CAD build for the part. Positions are in the model's coordinates, mm. Face numbers are marked on the shaded views. Round coordinates to 2 decimals unless told otherwise and drop trailing zeros. Loops run counter-clockwise (first coordinate to the right, second up) from the corner with the lowest first, then second, coordinate; pieces in that order, holes last.
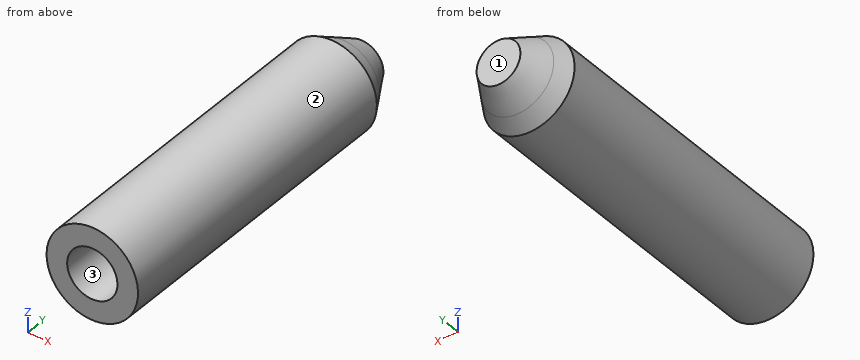
from build123d import *


with BuildPart() as f1:
    # F0 (on Right) → F1 (revolve)
    with BuildSketch(Plane.YZ):
        Polygon((35.489637, 5), (0, 5), (0, 2.75), (36.5, 2.75), (37.221688, 4), align=None)
        Polygon((40, 2.395941), (37.221688, 4), (36.5, 2.75), (38.087713, 0), (40, 0), align=None)
    revolve(axis=Axis((0, 39.043857, 0), (0, -1, 0)))


solid = f1.part
Item 1: Mould opens along X. For the marked faces 1, 2 and 3 say: released by +X, released by -X, zero draft, split by the parting line, or undercut.
Verdict:
face 1: zero draft
face 2: split by the parting line
face 3: undercut
Item 2: Cut at A-A (y = 3). List the corners of the cut face in (x, z).
Verdict:
outline: circle Ø10 at (0, 0); hole circle Ø5.5 at (0, 0)
Item 3: Flat gauge pins, fed straight in: P1, Ø1.5, axis at x = -1, z = 1.5, coming from the -Y side; P2, Ø6, axis at x = -1, y = 33.5, coming from the -Z side; P3, Ø3, axis at x = 3.5, y = 4, coming from the -Z side; P4, Ø2, axis at x = 1.5, y = 21, coming from the +Z side. Where does each tip first touch, or does it go through?
Verdict:
P1: stops at y = 36.61
P2: stops at z = -5
P3: stops at z = -4.58
P4: stops at z = 4.97
Item 4: Wall check: L1, parallel to X at y = 8.5, z = 0; L2, parallel to Z at x = 3, y = 16. Give the ranges that are in metal, low to high.
Verdict:
L1: x = -5 to -2.75, 2.75 to 5
L2: z = -4 to 4
